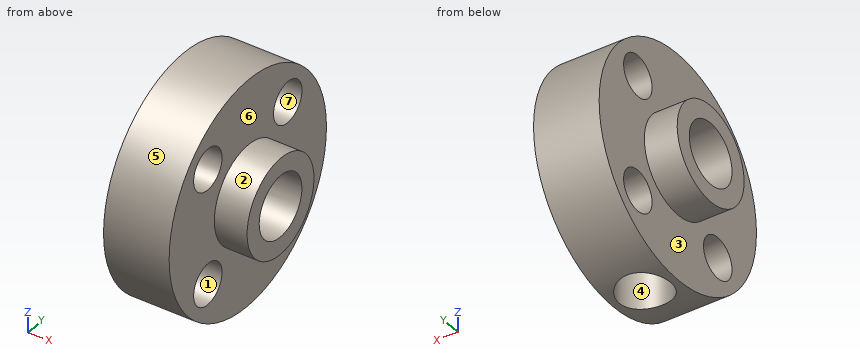
```python
from build123d import *

# Parameters (mm, degrees)
ESQUISSE2_R                  = 3
ENL_V_MAT_EXTRU_1_DEPTH      = 13.7
ESQUISSE3_R                  = 2
ENL_V_MAT_EXTRU_2_DEPTH      = 10
R_P_TITION_CIRCULAIRE1_COUNT = 4
ESQUISSE5_R                  = 2.5
ENL_V_MAT_EXTRU_3_DEPTH      = 12.05


with BuildPart() as part:
    # Esquisse1 → Révolution1 (revolve)
    with BuildSketch(Plane(origin=(0, 0, 0), x_dir=(1, 0, 0), z_dir=(0, 1, 0))):
        Polygon((-40.200130208, 0), (-40.200130208, 4.7), (-37.020130208, 4.7), (-37.020130208, 11.05), (-30.670130208, 11.05), (-30.670130208, 4.7), (-27.500130208, 4.7), (-27.500130208, 0), align=None)
    revolve(axis=Axis((-53.297005208, 0, 0), (1, 0, 0)))

    # Esquisse2 → Enlèv. mat.-Extru.1 (cut, through all)
    with BuildSketch(Plane.ZY.offset(40.200130208)):
        Circle(ESQUISSE2_R)
    extrude(amount=-ENL_V_MAT_EXTRU_1_DEPTH, mode=Mode.SUBTRACT)

    # Esquisse3 → Enlèv. mat.-Extru.2 (cut)
    with BuildSketch(Plane.ZY.offset(37.020130208)):
        with Locations((-5.614427843, 5.614427843)):
            Circle(ESQUISSE3_R)
    enl_v_mat_extru_2 = extrude(amount=-ENL_V_MAT_EXTRU_2_DEPTH, mode=Mode.SUBTRACT)

    # Répétition circulaire1: Enlèv. mat.-Extru.2 ×4 about axis
    r_p_tition_circulaire1_axis = Axis((0, 0, 0), (1, 0, 0))
    for i in range(1, R_P_TITION_CIRCULAIRE1_COUNT):
        add(enl_v_mat_extru_2.rotate(r_p_tition_circulaire1_axis, i * 360 / R_P_TITION_CIRCULAIRE1_COUNT), mode=Mode.SUBTRACT)

    # Esquisse5 → Enlèv. mat.-Extru.3 (cut, through all)
    with BuildSketch(Plane.XY):
        with Locations((-33.845130208, 0)):
            Circle(ESQUISSE5_R)
    extrude(amount=-ENL_V_MAT_EXTRU_3_DEPTH, mode=Mode.SUBTRACT)


solid = part.part
```
Geometry: final body of the model. Coordinates: model frame, mm. Face numbers are marked on the shaded views. A direction names the side the tool comes from. Coordinates: 2 decimals unless noted, no trailing zeros. Order: outer loops, then holes, each group sorted by start corner. A loop starts at its lowest first (then second) coordinate and runs counter-clockwise, first axis right, second up.
Item 1: Section query A-A (z = 0). Output: boundary loops of the cut face in (x, y).
Answer:
outline: (-40.2, -4.7) - (-37.02, -4.7) - (-37.02, -11.05) - (-30.67, -11.05) - (-30.67, -4.7) - (-27.5, -4.7) - (-27.5, -3) - (-40.2, -3) - close; (-40.2, 3) - (-27.5, 3) - (-27.5, 4.7) - (-30.67, 4.7) - (-30.67, 11.05) - (-37.02, 11.05) - (-37.02, 4.7) - (-40.2, 4.7) - close
Item 2: Contact query for flat-ended pins moving along their axis: P1, Ø5, axis at y = 5.61, z = 5.61, coming from the +X side; P2, Ø2, axis at x = -30.5, y = -6, coming from the +Z side; P3, Ø5, axis at x = -31.5, y = 7.5, coming from the +Z side. Output: stop coordinate, or through.
Answer:
P1: stops at x = -30.67
P2: stops at z = 9.85
P3: stops at z = 9.85
Item 3: Section query D-D (x = -34). Output: boundary loops of the cut face in (y, z), then the cut area to 3 significant figures.
Answer:
outline: (-2.5, -10.76) - (-2.5, -1.67) arc R3 cw (long way) to (2.5, -1.67) - (2.5, -10.76) arc R11.05 ccw (long way) to start; hole circle Ø4 at (-5.61, -5.61); hole circle Ø4 at (-5.61, 5.61); hole circle Ø4 at (5.61, -5.61); hole circle Ø4 at (5.61, 5.61)
area: 263 mm2
Item 4: Section query C-C (z = 4). Output: boundary loops of the cut face in (x, y).
Answer:
outline: (-40.2, -2.47) - (-37.02, -2.47) - (-37.02, -4.43) - (-30.67, -4.43) - (-30.67, -2.47) - (-27.5, -2.47) - (-27.5, 2.47) - (-30.67, 2.47) - (-30.67, 4.43) - (-37.02, 4.43) - (-37.02, 2.47) - (-40.2, 2.47) - close; (-37.02, -10.3) - (-30.67, -10.3) - (-30.67, -6.79) - (-37.02, -6.79) - close; (-37.02, 6.79) - (-30.67, 6.79) - (-30.67, 10.3) - (-37.02, 10.3) - close
Item 5: Draft query along Z for the marked faces 5, 6 and 7. Return one class per face: released by +Z, released by -Z, zero draft, split by the parting line, or undercut.
Answer:
face 5: split by the parting line
face 6: zero draft
face 7: undercut
Item 6: Material intervals for line 1 along X through (y, z) = (0, -7.25); line 2 along Y through (x, z) = (-32.75, 0); line 3 along Z through (x, y) = (-36.25, 4.25), sorted ascending.
Answer:
line 1: x = -37.02 to -36.35, -31.35 to -30.67
line 2: y = -11.05 to -3, 3 to 11.05
line 3: z = -10.2 to -7.08, -4.15 to 4.15, 7.08 to 10.2
Item 7: Section query B-B (y = 6.5). Output: boundary loops of the cut face in (x, z).
Answer:
outline: (-37.02, -8.94) - (-30.67, -8.94) - (-30.67, -7.41) - (-37.02, -7.41) - close; (-37.02, -3.82) - (-30.67, -3.82) - (-30.67, 3.82) - (-37.02, 3.82) - close; (-37.02, 7.41) - (-30.67, 7.41) - (-30.67, 8.94) - (-37.02, 8.94) - close
Item 8: Access query for the marked faces 1, 2, 3 and 4. Directions: +Z, -Z, +X, -X, +Y, -Y. A direction counts if a zero-diameter tool reaches every point of the face in a straight line with its end or side. Return the directions, or none.
Answer:
face 1: +X, -X
face 2: +X
face 3: -X
face 4: -Z
